Could you check a few things on this model? Use its own coordinates, in mm. A direction names the side the tool comes from. Round coordinates to 2 decimals unless told otherwise and drop trailing zeros. Write each loop counter-clockwise with the first axis right and the second up, starting at its lowest first coordinate (ties: lowest second). Pieces come first, ordered by that corner, then holes. Notation, with made-up numbers: M -19.75,54 L -12.75,54 A6 ccw -12.75,62 Z; hole C -17,54.5 d2. An arc over 180 degrees is marked long. One line per item, written item: value. Start each with the question number.
(1) Which directions (+Z, -Z, +X, -X, +Y, -Y) give clear straight access to the entire face, cutting with the end or side of a thin tool? Please do faces 1 (the face through (-8.75, 18, 4)), 2 (the face through (-9, 9, 4.5)), 3 (the face through (18, -8.75, 4)), 4 (the face through (18, 8.75, 4)).
(2) Thinking about a two-plate mould opening in Y: for faces 5 (the face through (7.25, -15, 4)), 6 (the face through (10.144, -10.184, 3.802)), 7 (the face through (-8.75, -18, 4)), which applies, released by +Y, released by -Y, zero draft, split by the parting line, or undercut?
(3) I'm going to push flat-ended pins straight in: pin 1 Ø0.5 at (x, y) = (9, 9) entering from +Z; pin 2 Ø4 at (y, z) = (-16.5, 2.5) entering from -X; pin 3 Ø1 at (x, z) = (-13.5, 2) entering from -Y. Where does each tip first touch, or does it pass through?
(4) I want a section at D-D on z = 6.5. Count the separate pieces of the cut face and the enclosed holes in it, and give its area (3 significant figures).
(5) I want a section at A-A on z = 3.25. Please give me the cut outline in (x, y).
(6) If I drill on L1, parallel to X at y = 14, z = 7.25; L2, parallel to Y at x = 3.5, z = 5.5, over which ranges is the centre line in solid material (lowest first)?
(7) I want a section at C-C on x = 0. Please give me the cut outline in (y, z).
(8) I want a section at B-B on y = 6. Please give me the cut outline in (x, z), and give its area (3 significant figures).
```python
from build123d import *

# Parameters (mm, degrees)
F1_DEPTH  = 7.5
F2_T      = -1.5
F4_DEPTH  = 7.5
F6_DEPTH  = 3
F7_R      = 3.25
F8_DEPTH  = 50.001
F9_R      = 3.25
F10_DEPTH = 50.001


with BuildPart() as f1:
    # F0 (on Top) → F1 (new body)
    with BuildSketch(Plane.XY):
        Polygon((25, -8.75), (25, 8.75), (8.75, 8.75), (8.75, 25), (-8.75, 25), (-8.75, 8.75), (-25, 8.75), (-25, -8.75), (-8.75, -8.75), (-8.75, -25), (8.75, -25), (8.75, -8.75), align=None)
    extrude(amount=F1_DEPTH)

    # F2
    f2_openings = [f1.faces().sort_by_distance(p)[0] for p in [
        (0, 0, 7.5),
    ]]
    offset(amount=F2_T, openings=f2_openings, kind=Kind.INTERSECTION)

    # F3 (on face) → F4 (join, through all)
    with BuildSketch(Plane.XY.offset(7.5)):
        Polygon((-8.75, 11.5784271247), (-11.5784271247, 8.75), (-8.75, 8.75), align=None)
        Polygon((8.75, 11.5784271247), (8.75, 8.75), (11.5784271247, 8.75), align=None)
        Polygon((-8.75, -11.5784271247), (-8.75, -8.75), (-11.5784271247, -8.75), align=None)
        Polygon((11.5784271247, -8.75), (8.75, -8.75), (8.75, -11.5784271247), align=None)
    extrude(amount=-F4_DEPTH)

    # F5 (on face) → F6 (cut)
    with BuildSketch(Plane.XY.offset(7.5)):
        with BuildLine():
            ThreePointArc((-9.6338834765, 9.6338834765), (-9.3905659649, 8.4106437412), (-8.3535533906, 9.1035533906))
            ThreePointArc((-8.3535533906, 9.1035533906), (-8.8165408163, 9.79646304), (-9.6338834765, 9.6338834765))
        make_face()
        with BuildLine():
            ThreePointArc((9.6338834765, 9.6338834765), (8.4106437412, 8.8165408163), (9.8535533906, 9.1035533906))
            ThreePointArc((9.8535533906, 9.1035533906), (9.79646304, 9.3905659649), (9.6338834765, 9.6338834765))
        make_face()
        with BuildLine():
            ThreePointArc((9.6338834765, -9.6338834765), (9.79646304, -9.3905659649), (9.8535533906, -9.1035533906))
            ThreePointArc((9.8535533906, -9.1035533906), (8.4106437412, -8.8165408163), (9.6338834765, -9.6338834765))
        make_face()
        with BuildLine():
            ThreePointArc((-9.6338834765, -9.6338834765), (-8.8165408163, -9.79646304), (-8.3535533906, -9.1035533906))
            ThreePointArc((-8.3535533906, -9.1035533906), (-9.3905659649, -8.4106437412), (-9.6338834765, -9.6338834765))
        make_face()
    extrude(amount=-F6_DEPTH, mode=Mode.SUBTRACT)

    # F7 (on face) → F8 (cut, through all)
    with BuildSketch(Plane.XZ.offset(25)):
        with Locations((0, 7.5)):
            Circle(F7_R)
    extrude(amount=-F8_DEPTH, mode=Mode.SUBTRACT)

    # F9 (on face) → F10 (cut, through all)
    with BuildSketch(Plane(origin=(-25, 0, 0), x_dir=(0, -1, 0), z_dir=(-1, 0, 0))):
        with Locations((0, 7.5)):
            Circle(F9_R)
    extrude(amount=-F10_DEPTH, mode=Mode.SUBTRACT)


solid = f1.part
```
Found:
1. face 1: +Z, -Z, -X, +Y
1. face 2: +Z
1. face 3: +Z, -Z, +X, -Y
1. face 4: +Z, -Z, +X, +Y
2. face 5: undercut
2. face 6: released by -Y
2. face 7: zero draft
3. pin 1: stops at z = 4.5
3. pin 2: stops at x = -8.75
3. pin 3: stops at y = -8.75
4. separate pieces: 4
4. enclosed holes: 4
4. area: 263 mm²
5. outline: M -25,-8.75 L -11.58,-8.75 L -8.75,-11.58 L -8.75,-25 L 8.75,-25 L 8.75,-11.58 L 11.58,-8.75 L 25,-8.75 L 25,8.75 L 11.58,8.75 L 8.75,11.58 L 8.75,25 L -8.75,25 L -8.75,11.58 L -11.58,8.75 L -25,8.75 Z; hole M -23.5,-7.25 L -7.25,-7.25 L -7.25,-23.5 L 7.25,-23.5 L 7.25,-7.25 L 23.5,-7.25 L 23.5,7.25 L 7.25,7.25 L 7.25,23.5 L -7.25,23.5 L -7.25,7.25 L -23.5,7.25 Z
6. L1: x = -8.75 to -7.25, 7.25 to 8.75
6. L2: y = -25 to -23.5, 23.5 to 25
7. outline: M -25,0 L 25,0 L 25,4.25 L 23.5,4.25 L 23.5,1.5 L -23.5,1.5 L -23.5,4.25 L -25,4.25 Z
8. outline: M -25,0 L 25,0 L 25,7.5 L 23.5,7.5 L 23.5,1.5 L -23.5,1.5 L -23.5,7.5 L -25,7.5 Z
8. area: 93.0 mm²
